Print and shaded views of the part. All mm, measured from the part's lowest x, y and z. A direction names the side the tool comes from. Give positions to 0.01 mm unless a question says otherwise; leave off trailing zeros. Order: outer loops, then holes, each group sorted by start corner. A loop starts at its lowest first (then second) coordinate and runs counter-clockwise, first axis right, second up. Notation, with made-up numbers: (69, 59.5) - (120, 59.5) arc R26 cw to (120, 82.5) - close; hole circle Ø6 at (76.5, -15.75). An arc over 180 degrees is marked (long way). Answer in a Markdown table with one row per item.
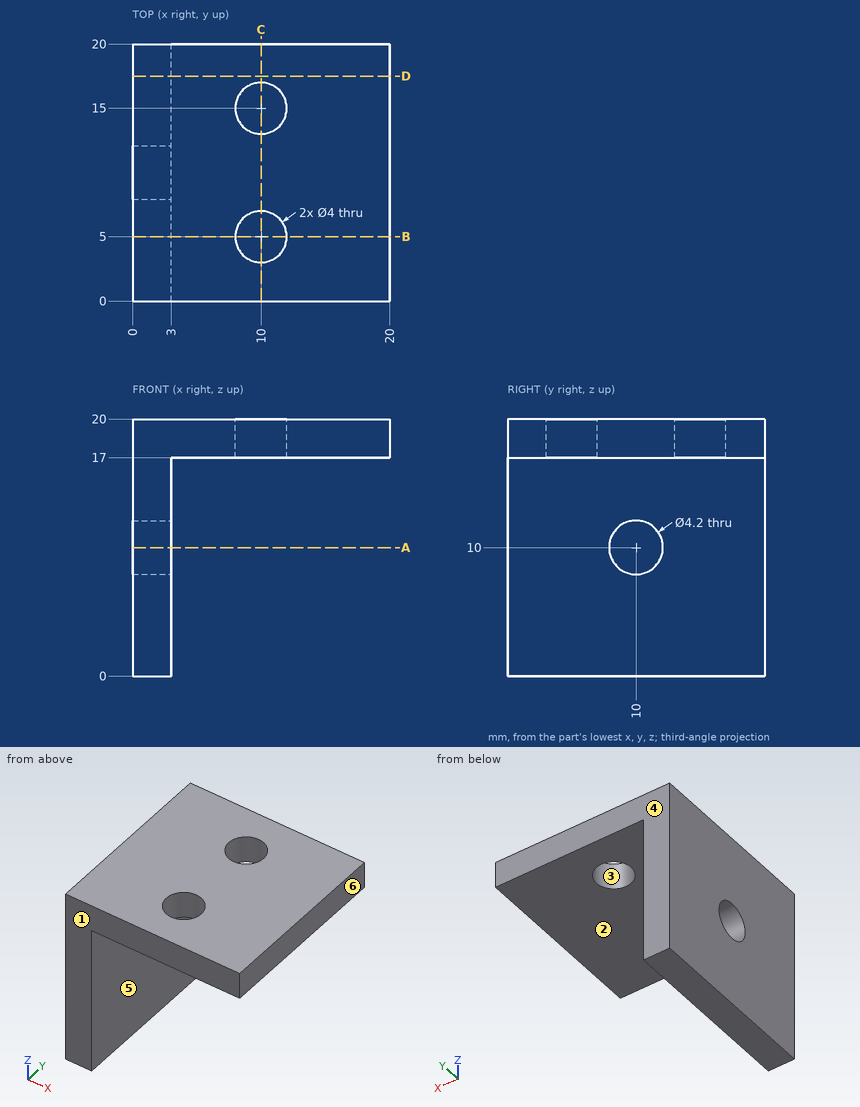
1. Cut at C-C on x = 10. Write the cut outline in (y, z).
Check result:
| item | result |
|---|---|
| outline | (0, 17) - (3, 17) - (3, 20) - (0, 20) - close; (7, 17) - (13, 17) - (13, 20) - (7, 20) - close; (17, 17) - (20, 17) - (20, 20) - (17, 20) - close |
2. Cut at D-D on y = 17.5. Write the cut outline in (x, z), and give its area (3 significant figures).
Check result:
| item | result |
|---|---|
| outline | (0, 0) - (3, 0) - (3, 17) - (20, 17) - (20, 20) - (0, 20) - close |
| area | 111 mm² |
3. Probe line 1 (Y direction, x = 10, z = 18.25); line 2 (Y direction, x = 1.05, z = 10); line 3 (Z direction, x = 16.5, y = 17.25). List the from-to ranges inside material, lowest first.
Check result:
| item | result |
|---|---|
| line 1 | y = 0 to 3, 7 to 13, 17 to 20 |
| line 2 | y = 0 to 7.9, 12.1 to 20 |
| line 3 | z = 17 to 20 |
4. Drop flat-ended pins along their axis: P1, Ø8.5, axis at x = 9, y = 8.5, coming from the -Z side; P2, Ø5, axis at y = 12, z = 9.5, coming from the +X side. Give the stop position or say it passes through.
Check result:
| item | result |
|---|---|
| P1 | stops at z = 17 |
| P2 | stops at x = 3 |
5. Which spindle directions (+Z, -Z, +X, -X, +Y, -Y) get a long thin tool onto all of the face, cutting with end or side? Do the marked faces 5 and 6. Say none if no direction does.
Check result:
| item | result |
|---|---|
| face 5 | -Z, +X, +Y, -Y |
| face 6 | +Z, -Z, +X, +Y, -Y |
6. Cut at B-B on y = 5. Write the cut outline in (x, z), and give its area (3 significant figures).
Check result:
| item | result |
|---|---|
| outline | (0, 0) - (3, 0) - (3, 17) - (8, 17) - (8, 20) - (0, 20) - close; (12, 17) - (20, 17) - (20, 20) - (12, 20) - close |
| area | 99.0 mm² |
7. Two-plate mould, pull along Y, no slides. Class the marked faces 1, 2, 3 and 4: +Y half, -Y half, draft (parallel to the pull), parting line (faces both ways), or undercut.
Check result:
| item | result |
|---|---|
| face 1 | -Y half |
| face 2 | draft |
| face 3 | undercut |
| face 4 | +Y half |
8. Cut at A-A on z = 10. Write the cut outline in (x, y), and give its area (3 significant figures).
Check result:
| item | result |
|---|---|
| outline | (0, 0) - (3, 0) - (3, 7.9) - (0, 7.9) - close; (0, 12.1) - (3, 12.1) - (3, 20) - (0, 20) - close |
| area | 47.4 mm² |
